Autodesk Inventor part; units mm, degrees
ref_plane "YZ Plane" through (0, 0, 0) normal (1, 0, 0) x (0, 1, 0)
ref_plane "XZ Plane" through (0, 0, 0) normal (0, 1, 0) x (-1, 0, 0)
ref_plane "XY Plane" through (0, 0, 0) normal (0, 0, 1) x (1, 0, 0)
sketch "Náčrt2" plane through (0, 0, 0) normal (1, 0, 0) x (0, 1, 0)
  circle A0 centre (0, 0) radius 6.5
  line L0 (31.5, 12.5) -> (0, 12.5)
  line L1 (31.5, 12.5) -> (31.5, 4.5)
  line L2 (31.5, 4.5) -> (6.4868, -10.6851)
  arc A1 (0, 12.5) -> (6.4868, -10.6851) centre (0, 0) ccw
  dimension "d0" = 13
  dimension "d1" = 6
  dimension "d2" = 31.5
  dimension "d3" = 8
extrude "Vysunutí1" add sketch "Náčrt2" along normal blind 30
fillet "Zaoblení1" radius 4 1 edges at (15, 31.5, 4.5)
chamfer "Zkosení1" distance 0.5 angle 45 2 edges at (0, -6.5, 0) (30, -6.5, 0)
properties part number "DD_KVD_003_10_A" material "Nerezová ocel"
Could you check a few things on this model? Use its own coordinates, in mm. Give positions to 0.01 mm unless a question says otherwise; leave off trailing zeros. Write each loop counter-clockwise with the first axis right and the second up, starting at its lowest first coordinate (ties: lowest second). Pieces come first, ordered by that corner, then holes. Notation, with made-up numbers: (-18.75, 87.5) - (-10.75, 87.5) arc R11 ccw to (-10.75, 106.5) - close; hole circle Ø6 at (81.25, -20.75). An arc over 180 degrees is marked (long way). Use CSV: the item, a comma, the result in double quotes. Start each with the question number.
Item 1: I'm going to push flat-ended pins straight in: pin 1 (1.5 mm diameter, centred on x = 22, y = 24, fed in from -Z); pin 2 (4 mm diameter, centred on x = 5, y = 3, fed in from -Z); pin 3 (6 mm diameter, centred on x = 27, y = 14, fed in from -Z). Where does each tip first touch, or does it pass through?
Item 2: I want a section at D-D, the plane z = 7.75. Please give me the cut outline in (x, y).
Item 3: I want a section at B-B, the plane x = 20. Please give me the cut outline in (y, z), then the cut area to 3 significant figures.
Item 4: If I drill on line 1 along Z through (x, y) = (8.25, 0); line 2 along Z through (x, y) = (24.5, 6); line 3 along Y through (x, z) = (12.25, 1.75), over which ranges is the centre line in solid material (lowest first)?
Item 5: I want a section at C-C, the plane y = 13.5. Please give me the cut outline in (x, z).
Item 6: I want a section at A-A, the plane z = 0. Please give me the cut outline in (x, y), then the cut area to 3 significant figures.
Findings:
1,pin 1,"stops at z = -0.51"
1,pin 2,"stops at z = -12.46"
1,pin 3,"stops at z = -7.95"
2,outline,"(0, -9.81) - (30, -9.81) - (30, 31.5) - (0, 31.5) - close"
3,outline,"(0, 12.5) arc R12.5 ccw (long way) to (6.49, -10.69) - (29.58, 3.33) arc R4 ccw to (31.5, 6.75) - (31.5, 12.5) - close; hole circle Ø13 at (0, 0)"
3,area,"660 mm2"
4,line 1,"z = -12.5 to -6.5, 6.5 to 12.5"
4,line 2,"z = -10.97 to -2.5, 2.5 to 12.5"
4,line 3,"y = -12.38 to -6.26, 6.26 to 26.97"
5,outline,"(0, -6.43) - (30, -6.43) - (30, 12.5) - (0, 12.5) - close"
6,outline,"(0, -12.5) - (30, -12.5) - (30, -7) - (29.5, -6.5) - (0.5, -6.5) - (0, -7) - close; (0, 7) - (0.5, 6.5) - (29.5, 6.5) - (30, 7) - (30, 24.09) - (0, 24.09) - close"
6,area,"707 mm2"
